from build123d import *

# Parameters (mm, degrees)
F0_W     = 101.6
F0_H     = 63.5
F1_DEPTH = 49.0601
F3_DEPTH = 63.501
F5_D     = 6.35


with BuildPart() as f1:
    # F0 (on Front) → F1 (new body, symmetric)
    with BuildSketch(Plane.XZ):
        with Locations((25.231418, -31.75)):
            Rectangle(F0_W, F0_H)
    extrude(amount=F1_DEPTH, both=True)

    # F2 (on face) → F3 (cut, through all)
    with BuildSketch(Plane.XY):
        with BuildLine():
            ThreePointArc((25.231418, -49.0601), (-10.689607, -34.181124), (-25.568582, 1.7399))
            Line((-25.568582, 1.7399), (-25.568582, -49.0601))
            Line((-25.568582, -49.0601), (25.231418, -49.0601))
        make_face()
        with BuildLine():
            Line((76.031418, -49.0601), (76.031418, 1.7399))
            ThreePointArc((76.031418, 1.7399), (61.152442, -34.181124), (25.231418, -49.0601))
            Line((25.231418, -49.0601), (76.031418, -49.0601))
        make_face()
    extrude(amount=-F3_DEPTH, mode=Mode.SUBTRACT)

    # F5 (through all)
    with Locations(Plane(origin=(0, 0, -63.5), x_dir=(1, 0, 0), z_dir=(0, 0, -1))):
        with Locations((25.231418, -1.7399)):
            Hole(F5_D / 2)


solid = f1.part
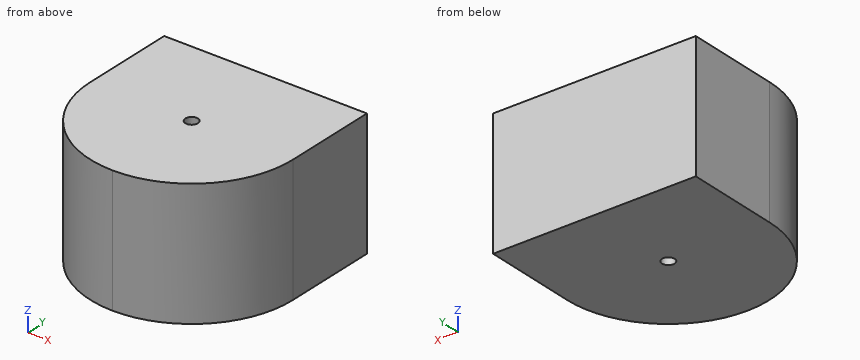
Work out the finished part from the listing and answer in its coordinate system (mm). Round coordinates to 2 decimals unless told otherwise and drop trailing zeros. Order: outer loops, then holes, each group sorted by start corner. A loop starts at its lowest first (then second) coordinate and runs counter-clockwise, first axis right, second up. Notation, with made-up numbers: M 87,84.5 L 107,84.5 A22 cw 107,92.5 Z; hole C 34.25,76 d1. An arc over 180 degrees is marked long. Put each result on its own line as item: value. Start each with the question number.
Q1. Section C-C, the plane y = -41 is taken. Write down the section's boundary in (x, z), and give its area (3 significant figures).
Q2. Section A-A, the plane z = -10 is taken. Write down the section's boundary in (x, y) (3 decimals).
Q3. Flat-ended cylindrical pins translate along their axes: pin 1 (12 mm diameter, centred on x = 57, z = -57, fed in from -Y); pin 2 (8 mm diameter, centred on x = 35.5, z = -20.5, fed in from -Y); pin 3 (8 mm diameter, centred on x = 46.5, z = -15, fed in from -Y). Find the tip coordinate at first contact, or state that the pin passes through.
Q4. Straight lines are drawn through the part: L1, parallel to Y at x = 24, z = -5.5; L2, parallel to X at y = -43, z = -17; L3, parallel to Y at x = 55, z = -58.5. For each, find the intervals that lie inside material, in ascending order. Write a range as [from, to].
Q5. Section B-B, the plane x = 10.5 is taken. Write down the section's boundary in (y, z).
Findings below:
1. outline: M -2.23,-63.5 L 52.69,-63.5 L 52.69,0 L -2.23,0 Z
1. area: 3,490 mm^2
2. outline: M -25.569,1.74 A50.8 ccw 25.231,-49.06 A50.8 ccw 76.031,1.74 L 76.031,49.06 L -25.569,49.06 Z; hole C 25.231,1.74 d6.35
3. pin 1: stops at y = -42.04
3. pin 2: stops at y = -48.67
3. pin 3: stops at y = -46.03
4. L1: y = [-49.05, -1.19], [4.67, 49.06]
4. L2: x = [1.17, 49.29]
4. L3: y = [-39.42, 49.06]
5. outline: M -46.88,-63.5 L 49.06,-63.5 L 49.06,0 L -46.88,0 Z
